Model file for the job. Use its own axes, mm. A direction names the side the tool comes from. Round coordinates to 2 decimals unless told otherwise and drop trailing zeros. Order: outer loops, then holes, each group sorted by start corner. A loop starts at its lowest first (then second) coordinate and runs counter-clockwise, first axis right, second up. Notation, with made-up numbers: (0.25, 89.5) - (21.25, 89.5) arc R16 cw to (21.25, 96.5) - close; hole circle Ø2 at (68.5, 59.5). An arc over 180 degrees is marked (long way). Answer as CSV lines item,"result". Start each with the question number.
1. Pin check, flat tips, straight feed: pin 1 Ø8 at (y, z) = (2.5, 11.5) entering from +X (3 decimals); pin 2 Ø2 at (y, z) = (-3.5, 12) entering from +X; pin 3 Ø3 at (y, z) = (2.5, 8) entering from +X; pin 4 Ø10 at (x, z) = (-6, 5.5) entering from +Y. Stop position of each tip, or through.
2. Band-saw the part on A-A on z = 3.75. List the corners of the cut face in (x, y).
3. 3-axis set-ups, long thin cutter, end or side, ignore diameter. For faces 1 (the face through (0, 0, 0)), 2 (the face through (4.174, -3.521, 19.902)): which of +Z, -Z, +X, -X, +Y, -Y reach the whole face in a straight line?
4. Wall check: line 1 along Y through (x, z) = (3.75, 20.5); line 2 along Z through (x, y) = (-0.5, -2.5); line 3 along Y through (x, z) = (-5, 5.75). Give the ranges that are in metal, low to high. Write a range as [from, to].
5. Pull direction Y, two halves, no side cores. Call faces 3 (the face through (-7.598, 5.826, 13.204)), 4 (the face through (-0.065, -5.746, 19.902)), 5 (the face through (8, 0, 10)): released by +Y, released by -Y, zero draft, split by the parting line, or undercut.
Autodesk Fusion 360 part; units mm, degrees
sketch "Sketch1" plane through (0, 0, 0) normal (0, 0, 1) x (1, 0, 0)
  circle A0 centre (0, 0) radius 6.15
  dimension "d1" = 12.3
ref_plane "WorkPlane1" through (0, 0, 10) normal (0, 0, 1) x (1, 0, 0)
sketch "Sketch2" plane through (0, 0, 10) normal (0, 0, 1) x (1, 0, 0)
  circle A0 centre (0, 0) radius 7.75
  dimension "d3" = 15.5
loft "Loft1" add profiles "Sketch2", "Sketch1" section 1 section 2
sketch "Sketch3" plane through (0, 0, 10) normal (0, 0, 1) x (1, 0, 0)
  circle A0 centre (0, 0) radius 7.75
  circle A1 centre (0, 0) radius 9.575
  dimension "d4" = 19.15
extrude "Extrude1" add sketch "Sketch3" along normal blind 6.5 contours A0 | A1
sketch "Sketch4" plane through (0, 0, 16.5) normal (0, 0, 1) x (1, 0, 0)
  circle A0 centre (0, 0) radius 9.575
  circle A1 centre (0, 0) radius 5.25 construction
  line L0 (0, 5.25) -> (0, -5.25) construction
  circle A2 centre (0, 5.25) radius 0.5
  circle A3 centre (-3.7123, 3.7123) radius 0.5
  circle A4 centre (-3.7123, -3.7123) radius 0.5
  circle A5 centre (0, -5.25) radius 0.5
  circle A6 centre (3.7123, -3.7123) radius 0.5
  circle A7 centre (3.7123, 3.7123) radius 0.5
  dimension "d7" = 10.5
  dimension "d8" = 1
  dimension "d10" = 360
extrude "Extrude2" add sketch "Sketch4" along normal blind 7.15 contours A2 | A3 | A4 | A5 | A6 | A7
chamfer "Chamfer1" distance 0.25 angle 45 6 edges at (3.2461, 3.5315, 23.65) (-0.4662, 5.0692, 23.65) (-4.1785, 3.5315, 23.65) (-4.1785, -3.8931, 23.65) (-0.4662, -5.4308, 23.65) (3.2461, -3.8931, 23.65)
Reply:
1,pin 1,"stops at x = 9.575"
1,pin 2,"stops at x = 9.24"
1,pin 3,"stops at x = 7.46"
1,pin 4,"stops at y = 8.78"
2,outline,"circle Ø13.5 at (0, 0)"
3,face 1,"-Z, +X, -X, +Y, -Y"
3,face 2,"+Z"
4,line 1,"y = [-4.21, -3.21], [3.21, 4.21]"
4,line 2,"z = [0, 16.5]"
4,line 3,"y = [-5, 5]"
5,face 3,"split by the parting line"
5,face 4,"undercut"
5,face 5,"zero draft"
